Design review of the part built by this model. Coordinates are the model's own, in mm. A direction names the side the tool comes from. Coordinates: 2 decimals unless noted, no trailing zeros. Loops run counter-clockwise (first coordinate to the right, second up) from the corner with the lowest first, then second, coordinate; pieces in that order, holes last. Notation, with made-up numbers: (23.25, 15) -> (74.25, 15) arc R22 cw to (74.25, 35) -> close; hole circle Ø8 at (52.25, -0.5). An arc over 180 degrees is marked (long way). Use CSV: the item, a comma, the result in double quotes.
```python
from build123d import *

# Parameters (mm, degrees)
SKETCH_R        = 2.25
PAD_DEPTH       = 5
SKETCH001_R     = 3
POCKET_DEPTH    = 2
SKETCH002_W     = 10
SKETCH002_H     = 100
PAD001_DEPTH    = 110
FILLET_R        = 4
SKETCH003_W     = 80
SKETCH003_H     = 5
POCKET001_DEPTH = 70.001
FILLET001_R     = 2


with BuildPart() as part:
    # Sketch (on XY_Plane of Origin) → Pad (new body)
    with BuildSketch(Plane.XY):
        Polygon((-55, 40), (-55, -30), (55, -30), (55, 40), (17.5, 40), (17.5, -9.659887), (-17.5, -9.659887), (-17.5, 40), align=None)
        with Locations((-37.5, 0)):
            Circle(SKETCH_R, mode=Mode.SUBTRACT)
        with Locations((37.5, 0)):
            Circle(SKETCH_R, mode=Mode.SUBTRACT)
        with Locations((-37.5, 14.09116)):
            Circle(SKETCH_R, mode=Mode.SUBTRACT)
        with Locations((37.5, 14.09116)):
            Circle(SKETCH_R, mode=Mode.SUBTRACT)
        with Locations((-37.5, -15.058182)):
            Circle(SKETCH_R, mode=Mode.SUBTRACT)
        with Locations((37.5, -15.058182)):
            Circle(SKETCH_R, mode=Mode.SUBTRACT)
        with Locations((-37.5, 28.008329)):
            Circle(SKETCH_R, mode=Mode.SUBTRACT)
        with Locations((37.5, 28.008329)):
            Circle(SKETCH_R, mode=Mode.SUBTRACT)
    extrude(amount=PAD_DEPTH)

    # Sketch001 (on XY_Plane of Origin) → Pocket (cut)
    with BuildSketch(Plane.XY):
        with Locations((-37.5, 14.09116)):
            Circle(SKETCH001_R)
        with Locations((-37.5, 0)):
            Circle(SKETCH001_R)
        with Locations((-37.5, -15.058182)):
            Circle(SKETCH001_R)
        with Locations((37.5, 14.09116)):
            Circle(SKETCH001_R)
        with Locations((37.5, 0)):
            Circle(SKETCH001_R)
        with Locations((37.5, -15.058182)):
            Circle(SKETCH001_R)
        with Locations((-37.5, 28.008329)):
            Circle(SKETCH001_R)
        with Locations((37.5, 28.008329)):
            Circle(SKETCH001_R)
    extrude(amount=POCKET_DEPTH, mode=Mode.SUBTRACT)

    # Sketch002 (on Face7 of Pocket) → Pad001 (join)
    with BuildSketch(Plane.YZ.offset(55)):
        with Locations((-25, -50)):
            Rectangle(SKETCH002_W, SKETCH002_H)
    extrude(amount=-PAD001_DEPTH)

    # Fillet
    fillet_edges = [part.edges().sort_by_distance(p)[0] for p in [
        (0, -20, 0),
    ]]
    fillet(fillet_edges, radius=FILLET_R)

    # Sketch003 (on Face22 of Fillet) → Pocket001 (cut, through all)
    with BuildSketch(Plane.XZ.offset(30)):
        with Locations((-1.180287, -53.94736)):
            Rectangle(SKETCH003_W, SKETCH003_H)
        with Locations((-1.180287, -40.150993)):
            Rectangle(SKETCH003_W, SKETCH003_H)
        with Locations((-1.180287, -71.923223)):
            Rectangle(SKETCH003_W, SKETCH003_H)
        with Locations((-1.180287, -89.899086)):
            Rectangle(SKETCH003_W, SKETCH003_H)
    extrude(amount=-POCKET001_DEPTH, mode=Mode.SUBTRACT)

    # Fillet001
    fillet001_edges = [part.edges().sort_by_distance(p)[0] for p in [
        (-55, -30, -47.5),
        (0, -30, 5),
        (0, -30, -100),
        (55, -30, -47.5),
        (-41.180287, -30, -53.94736),
        (-1.180287, -30, -56.44736),
        (38.819713, -30, -53.94736),
        (-1.180287, -30, -51.44736),
        (-41.180287, -30, -40.150993),
        (-1.180287, -30, -42.650993),
        (38.819713, -30, -40.150993),
        (-1.180287, -30, -37.650993),
        (-41.180287, -30, -71.923223),
        (-1.180287, -30, -74.423223),
        (38.819713, -30, -71.923223),
        (-1.180287, -30, -69.423223),
        (-41.180287, -30, -89.899086),
        (-1.180287, -30, -92.399086),
        (38.819713, -30, -89.899086),
        (-1.180287, -30, -87.399086),
    ]]
    fillet(fillet001_edges, radius=FILLET001_R)


solid = part.part
```
Item 1: Add section A-A (x = 5). State how many separate pieces and enclosed holes the cut face has, then the cut area to 3 significant figures.
Checked values:
separate pieces,"5"
enclosed holes,"0"
area,"897 mm^2"
Item 2: To check wall thickness, follow line 1 along Y through (x, z) = (37.5, 0.9); line 2 along Z through (x, y) = (-41, -4); line 3 along Y through (x, z) = (-23, -11). State the ranges of each line that lie inside material, in increasing order.
Checked values:
line 1,"-30 to -18.06, -12.06 to -3, 3 to 11.09, 17.09 to 25.01, 31.01 to 40"
line 2,"0 to 5"
line 3,"-30 to -20"
Item 3: Clearance check with flat-ended pins moving along their axes: pin 1 (8 mm diameter, centred on x = 37.5, y = 14.09, fed in from -Z); pin 2 (12 mm diameter, centred on x = -16, y = -12.5, fed in from -Z); pin 3 (3 mm diameter, centred on x = 37, y = -1, fed in from -Z). State where each tip first meets the part, or that it passes through.
Checked values:
pin 1,"z = 0"
pin 2,"z = -0.88"
pin 3,"z = 2"
Item 4: Add section B-B (y = -25). Give the boundary of the cut face in (x, z).
Checked values:
outline,"(-55, -100) -> (55, -100) -> (55, 5) -> (-55, 5) -> close; hole (-41.18, -92.4) -> (38.82, -92.4) -> (38.82, -87.4) -> (-41.18, -87.4) -> close; hole (-41.18, -74.42) -> (38.82, -74.42) -> (38.82, -69.42) -> (-41.18, -69.42) -> close; hole (-41.18, -56.45) -> (38.82, -56.45) -> (38.82, -51.45) -> (-41.18, -51.45) -> close; hole (-41.18, -42.65) -> (38.82, -42.65) -> (38.82, -37.65) -> (-41.18, -37.65) -> close"
Item 5: Draft analysis for pull direction X (two halves, no side actions). For faces 1 (the face through (38.538, 26.012, 3.479)), 2 (the face through (-47.777, -18.797, -1.141)), 3 (the face through (-55, -22, -36)), state which applies: pulls with the +X half, pulls with the -X half, needs draft (parallel to the pull), parting line crosses it, or undercut.
Checked values:
face 1,"undercut"
face 2,"needs draft"
face 3,"pulls with the -X half"
Item 6: Add section C-C (y = 0). Give the boundary of the cut face in (x, z).
Checked values:
outline,"(-55, 0) -> (-40.5, 0) -> (-40.5, 2) -> (-39.75, 2) -> (-39.75, 5) -> (-55, 5) -> close; (-35.25, 2) -> (-34.5, 2) -> (-34.5, 0) -> (-17.5, 0) -> (-17.5, 5) -> (-35.25, 5) -> close; (17.5, 0) -> (34.5, 0) -> (34.5, 2) -> (35.25, 2) -> (35.25, 5) -> (17.5, 5) -> close; (39.75, 2) -> (40.5, 2) -> (40.5, 0) -> (55, 0) -> (55, 5) -> (39.75, 5) -> close"
Item 7: Add section D-D (z = -24). Give the boundary of the cut face in (x, y), then the cut area to 3 significant figures.
Checked values:
outline,"(-55, -28) arc R2 ccw to (-53, -30) -> (53, -30) arc R2 ccw to (55, -28) -> (55, -20) -> (-55, -20) -> close"
area,"1,100 mm^2"
Item 8: Machinability: for faces 4 (the face through (-41.18, -24, -54)), 5 (the face through (34.5, 14.2, 1)), 6 (the face through (1, -20, -63)), which of the approach directions +Z, -Z, +X, -X, +Y, -Y give a long, thin tool a straight path to every point of the face, cutting with its end or side? Answer none if there is none.
Checked values:
face 4,"+Y, -Y"
face 5,"-Z"
face 6,"-Z, +X, -X, +Y"
